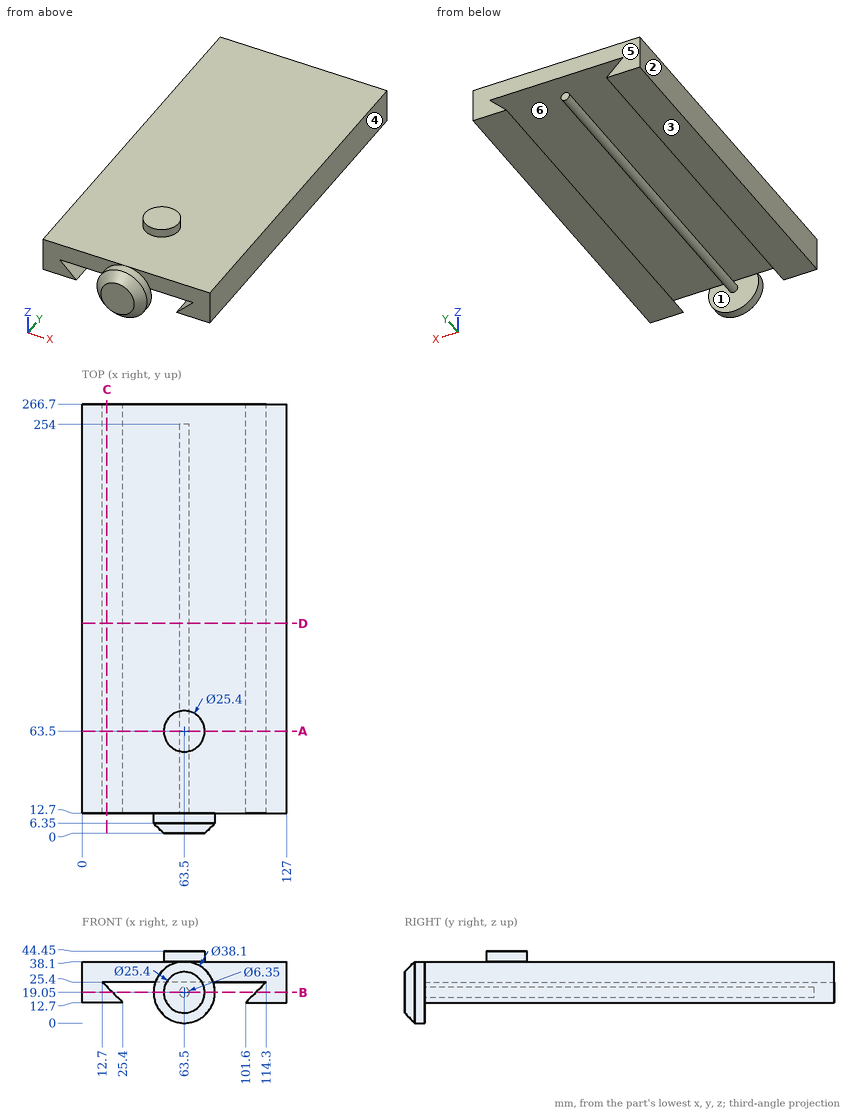
The drawing under review shows one solid part. Ordinate dimensions are in mm from its lowest x, y, z. A direction names the side the tool comes from. Give positions to 0.01 mm unless a question says otherwise; leave off trailing zeros. Write each loop counter-clockwise with the first axis right and the second up, starting at its lowest first coordinate (ties: lowest second). Pieces come first, ordered by that corner, then holes. Notation, with made-up numbers: (-34, 50) -> (1, 50) arc R33 cw to (1, 80) -> close; hole circle Ø7 at (40.5, 32.25). An arc over 180 degrees is marked (long way). Use CSV: the item, a comma, the result in double quotes.
Q1. Tool access review of the marked faces 5 and 6: name each direction out of +Z, -Z, +X, -X, +Y, -Y from which nothing blocks a thin tool from reaching the whole face with its end or side.
Conclusion:
face 5,"+Z, -Z, +X, -X, +Y"
face 6,"+Y"
Q2. Take a section at D-D, the plane y = 130.5. Write out the cut boundary in (x, z) (3 decimals).
Conclusion:
outline,"(0, 12.7) -> (25.4, 12.7) -> (12.7, 25.4) -> (114.3, 25.4) -> (101.6, 12.7) -> (127, 12.7) -> (127, 38.1) -> (0, 38.1) -> close; circle Ø6.35 at (63.5, 19.05)"
Q3. Mouldability with a two-part tool opening along X and no side actions: class the marked faces 1, 2, 3 and 4 as pulls with the +X half, pulls with the -X half, needs draft (parallel to the pull), parting line crosses it, or undercut.
Conclusion:
face 1,"undercut"
face 2,"pulls with the -X half"
face 3,"needs draft"
face 4,"pulls with the +X half"
Q4. Take a section at A-A, the plane y = 63.5. Write out the cut boundary in (x, z) (3 decimals), then the cut area to 3 significant figures.
Conclusion:
outline,"(0, 12.7) -> (25.4, 12.7) -> (12.7, 25.4) -> (114.3, 25.4) -> (101.6, 12.7) -> (127, 12.7) -> (127, 38.1) -> (76.2, 38.1) -> (76.2, 44.45) -> (50.8, 44.45) -> (50.8, 38.1) -> (0, 38.1) -> close; circle Ø6.35 at (63.5, 19.05)"
area,"2,290 mm2"
Q5. Take a section at C-C, the plane x = 15.5. Write out the cut boundary in (y, z), then the cut area to 3 significant figures.
Conclusion:
outline,"(12.7, 12.7) -> (266.7, 12.7) -> (266.7, 22.6) -> (12.7, 22.6) -> close; (12.7, 25.4) -> (266.7, 25.4) -> (266.7, 38.1) -> (12.7, 38.1) -> close"
area,"5,740 mm2"
Q6. Take a section at B-B, the plane z = 19.05. Write out the cut boundary in (x, y) (3 decimals).
Conclusion:
outline,"(0, 12.7) -> (19.05, 12.7) -> (19.05, 266.7) -> (0, 266.7) -> close; (44.45, 6.35) -> (50.8, 0) -> (76.2, 0) -> (82.55, 6.35) -> (82.55, 12.7) -> (66.675, 12.7) -> (66.675, 254) -> (60.325, 254) -> (60.325, 12.7) -> (44.45, 12.7) -> close; (107.95, 12.7) -> (127, 12.7) -> (127, 266.7) -> (107.95, 266.7) -> close"
Q7. To check wall thickness, follow probe 1 along X at (y, z) = (40, 18.5); probe 2 along Y at (x, z) = (85, 34.5); probe 3 along Z at (x, y) = (10, 101). State the ranges of each line that lie inside material, in increasing order. Write a range as [from, to].
Conclusion:
probe 1,"[0, 19.6], [60.37, 66.63], [107.4, 127]"
probe 2,"[12.7, 266.7]"
probe 3,"[12.7, 38.1]"
Q8. For P1, Ø20.5, axis at x = 10.5, y = 101, coming from the -Z side; P2, Ø12.5, axis at x = 68.5, z = 17, coming from the +Y side; P3, Ø8, axis at x = 81, y = 176, coming from the +Z side; P4, Ø12.5, axis at x = 46, z = 26, coming from the -Y side, all flat-tipped, find the tip position at first contact; note any pin that passes through.
Conclusion:
P1,"z = 12.7"
P2,"y = 254"
P3,"z = 38.1"
P4,"y = 0"
